Verification items for the finished model (mm, model axes). Coordinates: 2 decimals unless noted, no trailing zeros. Order: outer loops, then holes, each group sorted by start corner. A loop starts at its lowest first (then second) coordinate and runs counter-clockwise, first axis right, second up. Notation, with made-up numbers: M 3,11.5 L 16,11.5 A27 ccw 16,29.5 Z; hole C 13.5,40.25 d11. An arc over 180 degrees is marked long. Return JSON: item names as keys, results as strings. Group by question number.
Q1. Thickness scan on probe 1 along X at (y, z) = (-5, -6); probe 2 along X at (y, z) = (5.5, 7.5); probe 3 along Z at (x, y) = (858, 8.5). Record the ranges inside material, lowest first.
Q2. Go/stop test with flat-tipped pins: pin 1 Ø4 at (x, y) = (692.5, 2) entering from +Z; pin 2 Ø1 at (x, y) = (626.5, -5) entering from -Z; pin 3 Ø6 at (x, y) = (578, -6.5) entering from +Z; pin 4 Ø4 at (x, y) = (1060, 4) entering from +Z. Record where each tip stops, or that it passes through.
Q3. Section check B-B, the plane x = 133.5. Enter the section's corners in (y, z), then the cut area to 3 significant figures.
Q4. Section check A-A, the plane z = 0. Enter the section's corners in (x, y), then the cut area to 3 significant figures.
from build123d import *

# Parameters (mm, degrees)
SKETCH_1_R      = 10
EXTRUDE_1_DEPTH = 1500
SKETCH_2_R      = 5
EXTRUDE_3_DEPTH = 15
SKETCH_3_R      = 6
EXTRUDE_4_DEPTH = 40
EXTRUDE_START   = 15
SKETCH_4_R      = 5
EXTRUDE_5_DEPTH = 15
CHAMFER_4_SIZE  = 1
CHAMFER_5_SIZE  = 1


with BuildPart() as part:
    # Эскиз1 → Бобышка-Вытянуть1 (new body)
    with BuildSketch(Plane(origin=(0, 0, 0), x_dir=(0, 0, -1), z_dir=(1, 0, 0))):
        Circle(SKETCH_1_R)
    extrude(amount=EXTRUDE_1_DEPTH)

    # Эскиз2 → Бобышка-Вытянуть3 (add)
    with BuildSketch(Plane.ZY):
        with Locations(Location((0, 0, 0), (0, 0, 180))):
            Circle(SKETCH_2_R)
    extrude(amount=EXTRUDE_3_DEPTH)

    # Эскиз3 → Бобышка-Вытянуть4 (add)
    with BuildSketch(Plane(origin=(1500, 0, 0), x_dir=(0, 0, -1), z_dir=(1, 0, 0))):
        Circle(SKETCH_3_R)
    extrude(amount=EXTRUDE_4_DEPTH)

    # Эскиз4 → Бобышка-Вытянуть5 (add)
    with BuildSketch(Plane(origin=(1540, 0, 0), x_dir=(0, 0, -1), z_dir=(1, 0, 0)).offset(EXTRUDE_START)):
        Circle(SKETCH_4_R)
    extrude(amount=-EXTRUDE_5_DEPTH)

    # Фаска4
    chamfer_4_edges = [part.edges().sort_by_distance(p)[0] for p in [
        (1555, 0, 5),
        (1500, 0, 10),
    ]]
    chamfer(chamfer_4_edges, length=CHAMFER_4_SIZE)

    # Фаска5
    chamfer_5_edges = [part.edges().sort_by_distance(p)[0] for p in [
        (0, 0, 10),
        (-15, 0, 5),
    ]]
    chamfer(chamfer_5_edges, length=CHAMFER_5_SIZE)


solid = part.part
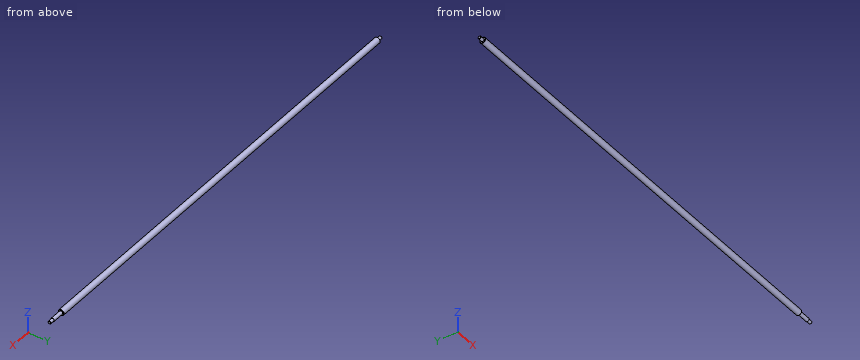
Numbers:
{
 "1": {"probe 1": "x = 0 to 1500", "probe 2": "x = 0.3 to 1499.7", "probe 3": "z = -5.27 to 5.27"},
 "2": {"pin 1": "stops at z = 10", "pin 2": "stops at z = -8.93", "pin 3": "stops at z = 9.37", "pin 4": "stops at z = 9.8"},
 "3": {"outline": "C 0,0 d20", "area": "314 mm2"},
 "4": {"outline": "M -15,-4 L -14,-5 L 0,-5 L 0,-9 L 1,-10 L 1499,-10 L 1500,-9 L 1500,-6 L 1540,-6 L 1540,-5 L 1554,-5 L 1555,-4 L 1555,4 L 1554,5 L 1540,5 L 1540,6 L 1500,6 L 1500,9 L 1499,10 L 1,10 L 0,9 L 0,5 L -14,5 L -15,4 Z", "area": "30,800 mm2"}
}
